Geometry check sheet. Reference: the model listing, model coordinates, mm. Round coordinates to 2 decimals unless told otherwise and drop trailing zeros. Write each loop counter-clockwise with the first axis right and the second up, starting at its lowest first coordinate (ties: lowest second). Pieces come first, ordered by that corner, then holes. Notation, with made-up numbers: M 49,63.25 L 102,63.25 A26 cw 102,84.25 Z; hole C 52.25,-29.5 d11. An arc over 180 degrees is marked long. Put each result on its own line as item: value. Start each with the question number.
(1) Material ranges on probe 1 along X at (y, z) = (-43.85, 23); probe 2 along X at (y, z) = (-42, 0); probe 3 along X at (y, z) = (-44.8, -25.5), recorded low to high.
(2) Gauge pin test, flat ends, axial feed: pin 1 (6 mm diameter, centred on x = -23, z = 39.84, fed in from -Y); pin 2 (6 mm diameter, centred on x = 26, z = 26, fed in from +Y); pin 3 (1 mm diameter, centred on y = -44, z = -18.5, fed in from -X); pin 4 (1 mm diameter, centred on x = 39.5, y = -44.5, fed in from -Z). Record the tip position at first contact, or that the pin passes through.
(3) Section check D-D on z = -23. Record the cut outline in (x, y).
(4) Section check C-C on y = -41.75. Count the separate pieces of the cut face and the enclosed holes in it, then the cut area to 3 significant figures.
(5) Mould release check, pull along Z, two halves, no side actions. Record for faces 1 (the cylindrical face through (36.64, -43.49, 22.86)), 2 (the cylindrical face through (20.641, -43.488, 37.674)), 3 (the flat face through (36, -46.25, 12)), 4 (the cylindrical face through (52.937, -43.488, -16.671)): pulls with the +Z half, pulls with the -Z half, needs draft (parallel to the pull), parting line crosses it, or undercut.
(6) Section check A-A on x = 0. Record the cut outline in (y, z), then the cut area to 3 significant figures.
(7) Section check B-B on z = 35. Record the cut outline in (x, y), then the cut area to 3 significant figures.
from build123d import *

# Parameters (mm, degrees)
STOCK_BATTERYPLATE_1_START       = -46.25
STOCK_BATTERYPLATE_1_OUTLINE_R   = 55.5
STOCK_BATTERYPLATE_1_OUTLINE_R_2 = 3.2
STOCK_BATTERYPLATE_1_OUTLINE_R_3 = 3.175
STOCK_BATTERYPLATE_1_DEPTH       = 5.60286881
CUT_EXTRUDE1_REACH               = 80.689
SKETCH1_R                        = 37.5


# Read off the part's stored shape, not the designer's step: Stock-batteryplate-1
with BuildPart() as part:
    # Stock-batteryplate-1 outline → Stock-batteryplate-1 (new body)
    with BuildSketch(Plane(origin=(0, 0, 0), x_dir=(1, 0, 0), z_dir=(0, 1, 0)).offset(STOCK_BATTERYPLATE_1_START)):
        Circle(STOCK_BATTERYPLATE_1_OUTLINE_R)
        with Locations((-23, -39.837168574)):
            Circle(STOCK_BATTERYPLATE_1_OUTLINE_R_2, mode=Mode.SUBTRACT)
        with Locations((-39.837168574, -23)):
            Circle(STOCK_BATTERYPLATE_1_OUTLINE_R_2, mode=Mode.SUBTRACT)
        with Locations((-14.849242405, -14.849242405)):
            Circle(STOCK_BATTERYPLATE_1_OUTLINE_R_2, mode=Mode.SUBTRACT)
        with Locations((23, -39.837168574)):
            Circle(STOCK_BATTERYPLATE_1_OUTLINE_R_2, mode=Mode.SUBTRACT)
        with Locations((14.849242405, -14.849242405)):
            Circle(STOCK_BATTERYPLATE_1_OUTLINE_R_2, mode=Mode.SUBTRACT)
        with Locations((39.837168574, -23)):
            Circle(STOCK_BATTERYPLATE_1_OUTLINE_R_2, mode=Mode.SUBTRACT)
        with Locations((-39.837168574, 23)):
            Circle(STOCK_BATTERYPLATE_1_OUTLINE_R_2, mode=Mode.SUBTRACT)
        with Locations((-14.849242405, 14.849242405)):
            Circle(STOCK_BATTERYPLATE_1_OUTLINE_R_2, mode=Mode.SUBTRACT)
        with Locations((-23, 39.837168574)):
            Circle(STOCK_BATTERYPLATE_1_OUTLINE_R_2, mode=Mode.SUBTRACT)
        Circle(STOCK_BATTERYPLATE_1_OUTLINE_R_3, mode=Mode.SUBTRACT)
        with Locations((14.849242405, 14.849242405)):
            Circle(STOCK_BATTERYPLATE_1_OUTLINE_R_2, mode=Mode.SUBTRACT)
        with Locations((39.837168574, 23)):
            Circle(STOCK_BATTERYPLATE_1_OUTLINE_R_2, mode=Mode.SUBTRACT)
        with Locations((23, 39.837168574)):
            Circle(STOCK_BATTERYPLATE_1_OUTLINE_R_2, mode=Mode.SUBTRACT)
    extrude(amount=STOCK_BATTERYPLATE_1_DEPTH)

    # Sketch1 → Cut-Extrude1 (cut, up to next)
    with BuildSketch(Plane(origin=(0, -40.64713119, 0), x_dir=(1, 0, 0), z_dir=(0, 1, 0)), mode=Mode.PRIVATE) as cut_extrude1_sk1:
        with Locations(Location((0, 0, 0), (0, 0, 270))):
            Circle(SKETCH1_R)
    cut_extrude1_tool1 = extrude(cut_extrude1_sk1.sketch, amount=-CUT_EXTRUDE1_REACH, mode=Mode.PRIVATE) & part.part
    add(cut_extrude1_tool1.solids().sort_by_distance((0, -40.647131, 0))[0], mode=Mode.SUBTRACT)


solid = part.part
Answers follow:
1. probe 1: x = -50.51 to -43.04, -36.64 to -29.62, 29.62 to 36.64, 43.04 to 50.51
1. probe 2: x = -55.5 to -37.5, 37.5 to 55.5
1. probe 3: x = -49.3 to -41.83, -37.84 to -27.5, 27.5 to 37.84, 41.83 to 49.3
2. pin 1: passes through
2. pin 2: stops at y = -40.65
2. pin 3: stops at x = -52.5
2. pin 4: stops at z = -39.49
3. outline: M -50.51,-46.25 L -43.04,-46.25 L -43.04,-40.65 L -50.51,-40.65 Z; M -36.64,-46.25 L -29.62,-46.25 L -29.62,-40.65 L -36.64,-40.65 Z; M 29.62,-46.25 L 36.64,-46.25 L 36.64,-40.65 L 29.62,-40.65 Z; M 43.04,-46.25 L 50.51,-46.25 L 50.51,-40.65 L 43.04,-40.65 Z
4. separate pieces: 1
4. enclosed holes: 9
4. area: 5,000 mm^2
5. face 1: undercut
5. face 2: undercut
5. face 3: needs draft
5. face 4: parting line crosses it
6. outline: M -46.25,-55.5 L -40.65,-55.5 L -40.65,-37.5 L -46.25,-37.5 Z; M -46.25,37.5 L -40.65,37.5 L -40.65,55.5 L -46.25,55.5 Z
6. area: 202 mm^2
7. outline: M -43.07,-46.25 L -13.46,-46.25 L -13.46,-40.65 L -43.07,-40.65 Z; M 13.46,-46.25 L 43.07,-46.25 L 43.07,-40.65 L 13.46,-40.65 Z
7. area: 332 mm^2
